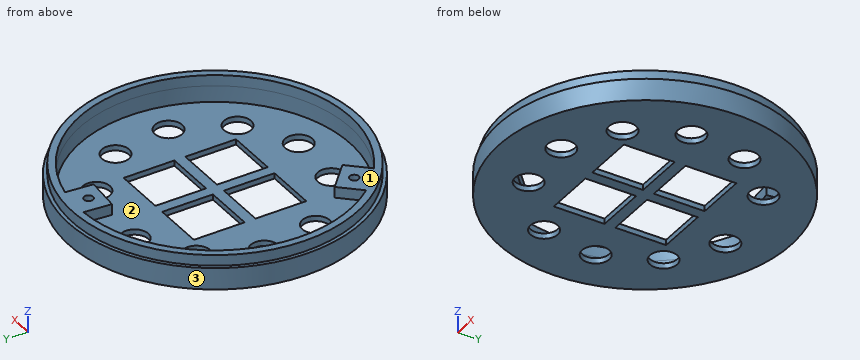
from build123d import *
from build123d.topology import SkipClean

# Parameters (mm, degrees)
SKETCH2_R           = 39.25
SKETCH2_R_2         = 1.25
BOSS_EXTRUDE1_DEPTH = 3
BOSS_EXTRUDE2_START = -6
SKETCH3_R           = 40.25
SKETCH3_R_2         = 37.25
SKETCH3_R_3         = 1.25
BOSS_EXTRUDE2_DEPTH = 6
SKETCH4_R           = 40.25
BOSS_EXTRUDE3_DEPTH = 1.5
SKETCH5_W           = 14
SKETCH5_H           = 14
CUT_EXTRUDE1_DEPTH  = 1.5
SKETCH7_R           = 3.75
CUT_EXTRUDE2_DEPTH  = 1.5


with BuildPart() as part:
    # Sketch2 → Boss-Extrude1 (new body)
    with BuildSketch(Plane(origin=(0, 0, 0), x_dir=(0, 1, 0), z_dir=(0, 0, 1))):
        with Locations(Location((0, 0, 0), (0, 0, 270))):
            Circle(SKETCH2_R)
        with BuildLine():
            Line((-18.29588, 23.55599), (-23.781033, 28.670978))
            ThreePointArc((-23.781033, 28.670978), (15.15094, 34.029568), (37.219306, 1.511877))
            Line((37.219306, 1.511877), (29.747846, 2.165545))
            Line((29.747846, 2.165545), (28.919866, -7.298305))
            Line((28.919866, -7.298305), (36.391326, -7.951973))
            ThreePointArc((36.391326, -7.951973), (-15.15094, -34.029568), (-30.260018, 21.723117))
            Line((-30.260018, 21.723117), (-24.774865, 16.60813))
            Line((-24.774865, 16.60813), (-18.29588, 23.55599))
        make_face(mode=Mode.SUBTRACT)
        with Locations(Location((-24.277949, 22.639554, 0), (0, 0, 270))):
            Circle(SKETCH2_R_2, mode=Mode.SUBTRACT)
        with Locations(Location((33.069586, -2.893214, 0), (0, 0, 270))):
            Circle(SKETCH2_R_2, mode=Mode.SUBTRACT)
    extrude(amount=BOSS_EXTRUDE1_DEPTH)

    # Sketch3 → Boss-Extrude2 (add)
    # profile 1 of 3: a face of its own
    with SkipClean():  # the faces are left unmerged after this step: merging them gives an invalid solid
        with BuildSketch(Plane.XY.offset(BOSS_EXTRUDE2_START)):
            with Locations(Location((0, 0, 0), (0, 0, 180))):
                Circle(SKETCH3_R)
            with Locations(Location((0, 0, 0), (0, 0, 219.67388))):
                Circle(SKETCH3_R_2, mode=Mode.SUBTRACT)
        # profile 2 of 3: a face of its own
        with BuildSketch(Plane.XY.offset(BOSS_EXTRUDE2_START)):
            with Locations((2.893214, 33.069586)):
                Circle(SKETCH3_R_3)
        # profile 3 of 3: a face of its own
        with BuildSketch(Plane.XY.offset(BOSS_EXTRUDE2_START)):
            with Locations((-22.639554, -24.277949)):
                Circle(SKETCH3_R_3)
        extrude(amount=BOSS_EXTRUDE2_DEPTH)


with BuildPart() as boss_extrude2_kept_piece:
    # of the separate pieces the step leaves, the one the design keeps (boss_extrude2_pieces_kept)
    add(part.part.solids().sort_by_distance((39.25, 0, 0))[0])

    # Sketch4 → Boss-Extrude3 (add)
    with SkipClean():  # the faces are left unmerged after this step: merging them gives an invalid solid
        with BuildSketch(Plane.XY.offset(-6)):
            with Locations(Location((0, 0, 0), (0, 0, 180))):
                Circle(SKETCH4_R)
        extrude(amount=BOSS_EXTRUDE3_DEPTH)

    # Sketch5 → Cut-Extrude1 (cut)
    with SkipClean():  # the faces are left unmerged after this step: merging them gives an invalid solid
        with BuildSketch(Plane(origin=(0, 0, -6), x_dir=(-1, 0, 0), z_dir=(0, 0, -1))):
            with Locations((-8.5, -8.5)):
                Rectangle(SKETCH5_W, SKETCH5_H)
            with Locations((-8.5, 8.5)):
                Rectangle(SKETCH5_W, SKETCH5_H)
            with Locations((8.5, 8.5)):
                Rectangle(SKETCH5_W, SKETCH5_H)
            with Locations((8.5, -8.5)):
                Rectangle(SKETCH5_W, SKETCH5_H)
        extrude(amount=-CUT_EXTRUDE1_DEPTH, mode=Mode.SUBTRACT)

    # Sketch7 → Cut-Extrude2 (cut)
    with SkipClean():  # the faces are left unmerged after this step: merging them gives an invalid solid
        with BuildSketch(Plane(origin=(0, 0, -6), x_dir=(-1, 0, 0), z_dir=(0, 0, -1))):
            with Locations((-25.126958, 11.736458)):
                Circle(SKETCH7_R)
            with Locations((-27.394136, -4.320851)):
                Circle(SKETCH7_R)
            with Locations((-20.294579, -18.900755)):
                Circle(SKETCH7_R)
            with Locations((-6.2558, -27.01802)):
                Circle(SKETCH7_R)
            with Locations((9.921992, -25.897153)):
                Circle(SKETCH7_R)
            with Locations((25.168506, -12.130508)):
                Circle(SKETCH7_R)
            with Locations((27.693803, 3.695429)):
                Circle(SKETCH7_R)
            with Locations((21.107164, 18.305479)):
                Circle(SKETCH7_R)
            with Locations((7.575753, 26.892581)):
                Circle(SKETCH7_R)
            with Locations((-14.268248, 23.780781)):
                Circle(SKETCH7_R)
        extrude(amount=-CUT_EXTRUDE2_DEPTH, mode=Mode.SUBTRACT)


solid = boss_extrude2_kept_piece.part
Work out the finished part from the listing and answer in its coordinate system (mm). Face numbers are marked on the shaded views. Coordinates: 2 decimals unless noted, no trailing zeros. Write each loop counter-clockwise with the first axis right and the second up, starting at its lowest first coordinate (ties: lowest second). Pieces come first, ordered by that corner, then holes. Notation, with made-up numbers: M 47.5,5 L 66.5,5 A13 ccw 66.5,17 Z; hole C 7.5,31 d5. An arc over 180 degrees is marked long. Write item = value, one per line.
1. The part is cut by section A-A (y = 16.5). Determine the outline of the cut face in (x, z), then the cut area to 3 significant figures.
Solution:
outline = M -36.71,-6 L -24.39,-6 L -24.39,-4.5 L -33.4,-4.5 L -33.4,3 L -35.61,3 L -35.61,0 L -36.71,0 Z; M -17.82,-6 L 36.71,-6 L 36.71,0 L 35.61,0 L 35.61,3 L 33.4,3 L 33.4,-4.5 L -17.82,-4.5 Z
area = 143 mm2
2. The part is cut by section B-B (z = -2.5). Determine the outline of the cut face in (x, y).
Solution:
outline = C 0,0 d80.5; hole C 0,0 d74.5
3. Straight lines are drawn through the part: line 1 (Z direction, x = -21, y = -24.5); line 2 (Y direction, x = 1, z = -1.75); line 3 (X direction, y = -34, z = -0.25). For each, find the intervals that lie inside material, in ascending order. Write a range as from..to.
Solution:
line_1 = -6..-4.5, 0..3
line_2 = -40.24..-37.24, 37.24..40.24
line_3 = -21.54..-15.22, 15.22..21.54
4. Flat-ended cylindrical pins translate along their axes: pin 1 (4 mm diameter, centred on x = -31.5, z = -3, fed in from +Y); pin 2 (0.8 mm diameter, centred on y = 5, z = -5.5, fed in from +X); pin 3 (8.5 mm diameter, centred on x = -27.69, y = 3.7, fed in from +Z). Find the tip coordinate at first contact, or state that the pin passes through.
Solution:
pin_1 = 27.38
pin_2 = 39.99
pin_3 = -4.5
5. Determine the mould class of the marked faces 1, 2 and 3 for opening direction X: released by +X, released by -X, zero draft, split by the parting line, or undercut.
Solution:
face_1 = zero draft
face_2 = undercut
face_3 = split by the parting line
6. The part is cut by section D-D (x = 33.5). Determine the outline of the cut face in (y, z), then the cut area to 3 significant figures.
Solution:
outline = M -22.31,-6 L 22.31,-6 L 22.31,0 L 20.45,0 L 20.45,3 L 16.29,3 L 16.29,-4.5 L -16.29,-4.5 L -16.29,3 L -20.45,3 L -20.45,0 L -22.31,0 Z
area = 146 mm2
7. The part is cut by section C-C (x = -9). Determine the outline of the cut face in (y, z), then the cut area to 3 significant figures.
Solution:
outline = M -39.23,-6 L -29.53,-6 L -29.53,-4.5 L -36.15,-4.5 L -36.15,3 L -38.2,3 L -38.2,0 L -39.23,0 Z; M -22.26,-6 L -15.5,-6 L -15.5,-4.5 L -22.26,-4.5 Z; M -1.5,-6 L 1.5,-6 L 1.5,-4.5 L -1.5,-4.5 Z; M 15.5,-6 L 23.42,-6 L 23.42,-4.5 L 15.5,-4.5 Z; M 30.36,-6 L 39.23,-6 L 39.23,0 L 38.2,0 L 38.2,3 L 36.15,3 L 36.15,-4.5 L 30.36,-4.5 Z
area = 94.5 mm2
